Design review of the part shown in the three views and the two pictorial views. Dimensions are in mm from the part's minimum x, y and z. A direction names the side the tool comes from. Coordinates: 2 decimals unless noted, no trailing zeros. Loops run counter-clockwise (first coordinate to the right, second up) from the corner with the lowest first, then second, coordinate; pieces in that order, holes last. Notation, with made-up numbers: (88, 76.25) -> (109, 76.25) arc R12 cw to (109, 91.25) -> close; hole circle Ø4 at (26.25, 64.5). An arc over 180 degrees is marked (long way). Answer in a Markdown table with one row per item.
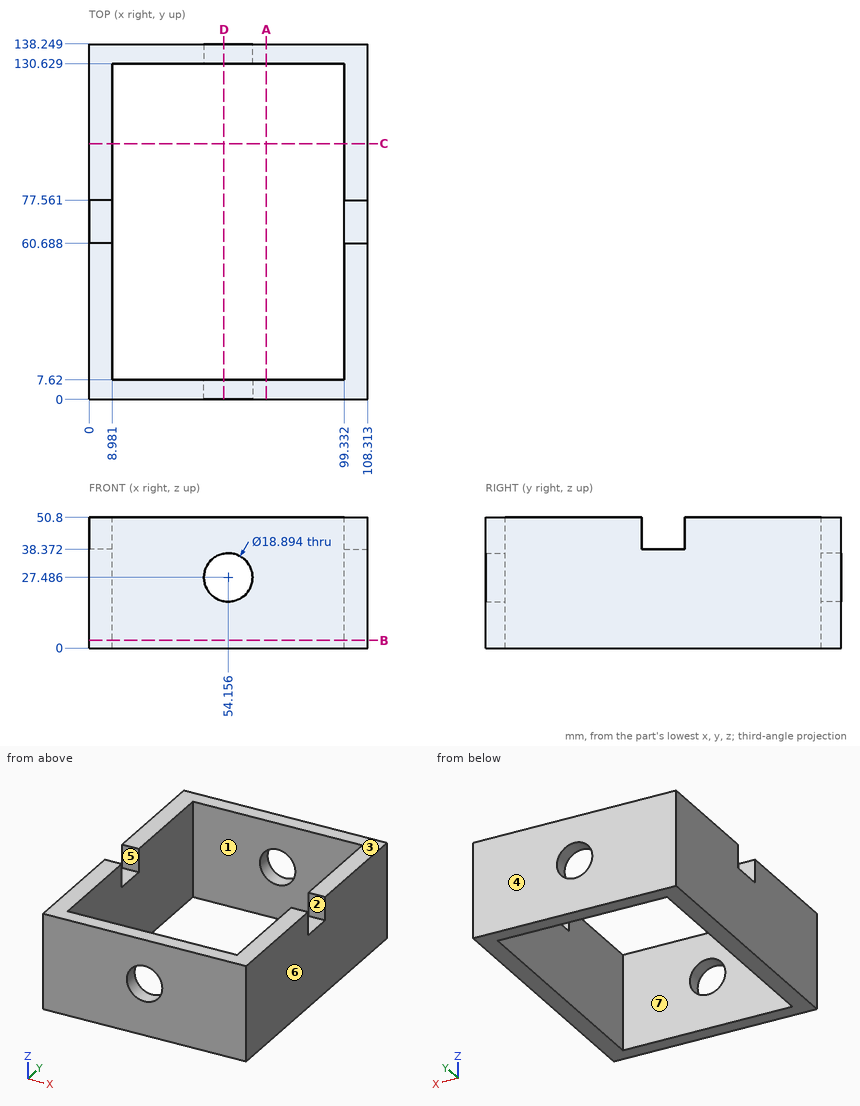
(1) To check wall thickness, follow probe 1 along X at (y, z) = (125.5, 13); probe 2 along Y at (x, z) = (51, 7); probe 3 along Y at (x, z) = (101, 39.5). State the ranges of each line that lie inside material, in increasing order.
Evaluation:
| item | result |
|---|---|
| probe 1 | x = 0 to 8.98, 99.33 to 108.31 |
| probe 2 | y = 0 to 7.62, 130.63 to 138.25 |
| probe 3 | y = 0 to 60.69, 77.56 to 138.25 |
(2) Tool access review of the marked faces 1, 2 and 3: name each direction out of +Z, -Z, +X, -X, +Y, -Y from which nothing blocks a thin tool from reaching the whole face with its end or side.
Evaluation:
| item | result |
|---|---|
| face 1 | +Z, -Z |
| face 2 | +Z, +X, -X |
| face 3 | +Z, +X, -X, +Y, -Y |
(3) Draft analysis for pull direction Y (two halves, no side actions). For the marked faces 4, 5, 6 and 7, state which applies: pulls with the +Y half, pulls with the -Y half, needs draft (parallel to the pull), parting line crosses it, or undercut.
Evaluation:
| item | result |
|---|---|
| face 4 | pulls with the +Y half |
| face 5 | undercut |
| face 6 | needs draft |
| face 7 | undercut |
(4) Take a section at C-C on y = 99.5. Give the boundary of the cut face in (x, z).
Evaluation:
| item | result |
|---|---|
| outline | (0, 0) -> (8.98, 0) -> (8.98, 50.8) -> (0, 50.8) -> close; (99.33, 0) -> (108.31, 0) -> (108.31, 50.8) -> (99.33, 50.8) -> close |
(5) Take a section at A-A on x = 69. Give the boundary of the cut face in (y, z), and give its area (3 significant figures).
Evaluation:
| item | result |
|---|---|
| outline | (0, 0) -> (7.62, 0) -> (7.62, 50.8) -> (0, 50.8) -> close; (130.63, 0) -> (138.25, 0) -> (138.25, 50.8) -> (130.63, 50.8) -> close |
| area | 774 mm² |
(6) Take a section at D-D on x = 52.5. Give the boundary of the cut face in (y, z) (1 decimal), and give its area (3 significant figures).
Evaluation:
| item | result |
|---|---|
| outline | (0, 0) -> (7.6, 0) -> (7.6, 18.2) -> (0, 18.2) -> close; (0, 36.8) -> (7.6, 36.8) -> (7.6, 50.8) -> (0, 50.8) -> close; (130.6, 0) -> (138.2, 0) -> (138.2, 18.2) -> (130.6, 18.2) -> close; (130.6, 36.8) -> (138.2, 36.8) -> (138.2, 50.8) -> (130.6, 50.8) -> close |
| area | 491 mm² |
(7) Take a section at B-B on z = 3. Give the boundary of the cut face in (x, y).
Evaluation:
| item | result |
|---|---|
| outline | (0, 0) -> (108.31, 0) -> (108.31, 138.25) -> (0, 138.25) -> close; hole (8.98, 7.62) -> (99.33, 7.62) -> (99.33, 130.63) -> (8.98, 130.63) -> close |
(8) For pin 1 (2.5 mm diameter, centred on x = 104.5, y = 73, fed in from +Z), flat-tipped, find the tip position at first contact; note if it passes through.
Evaluation:
| item | result |
|---|---|
| pin 1 | stops at z = 38.37 |
